Verification items for this drawing (mm, ordinates from the low corner). Round coordinates to 2 decimals unless told otherwise and drop trailing zeros. Loops run counter-clockwise (first coordinate to the right, second up) from the corner with the lowest first, then second, coordinate; pieces in that order, holes last. Notation, with made-up numbers: M -13,75 L -2,75 A24 ccw -2,104 Z; hole C -22,33.25 d11. An arc over 180 degrees is marked long. Write item = value, one per line.
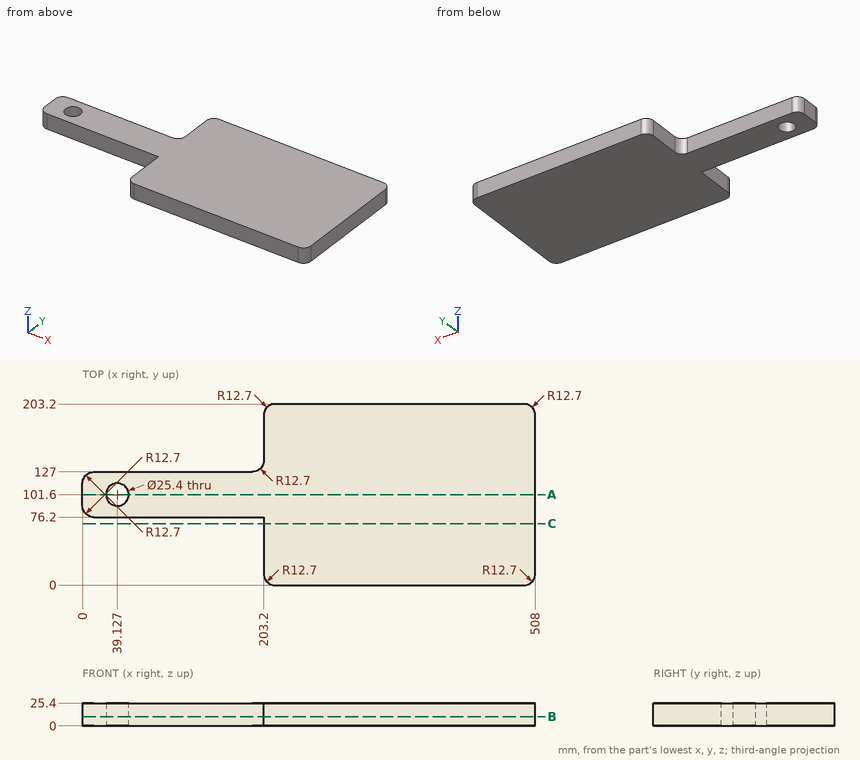
(1) Depth check by flat-ended pin: pin 1 Ø5 at (y, z) = (158, 13.5) entering from -X; pin 2 Ø3 at (x, z) = (148, 6) entering from -Y. Enter the tip coordinate at first touch or a pass-through.
Result set:
pin_1 = 203.2
pin_2 = 76.2
(2) Sectioned sample at B-B on z = 10.25. Record the cut outline in (x, y), then the cut area to 3 significant figures.
Result set:
outline = M 0,88.9 A12.7 ccw 12.7,76.2 L 203.2,76.2 L 203.2,12.7 A12.7 ccw 215.9,0 L 495.3,0 A12.7 ccw 508,12.7 L 508,190.5 A12.7 ccw 495.3,203.2 L 215.9,203.2 A12.7 ccw 203.2,190.5 L 203.2,139.7 A12.7 cw 190.5,127 L 12.7,127 A12.7 ccw 0,114.3 Z; hole C 39.13,101.6 d25.4
area = 71,600 mm2
(3) Sectioned sample at A-A on y = 101.6. Record the cut outline in (x, z), then the cut area to 3 significant figures.
Result set:
outline = M 0,0 L 26.43,0 L 26.43,25.4 L 0,25.4 Z; M 51.83,0 L 508,0 L 508,25.4 L 51.83,25.4 Z
area = 12,300 mm2
(4) Material ranges on line 1 along X through (y, z) = (22.5, 21); line 2 along Y through (x, z) = (177, 6.25); line 3 along X through (y, z) = (195, 12.5) (1 decimal), recorded low to high. Write a range as from..to.
Result set:
line_1 = 203.2..508
line_2 = 76.2..127
line_3 = 204..507.2
(5) Sectioned sample at C-C on y = 69. Record the cut outline in (x, z).
Result set:
outline = M 203.2,0 L 508,0 L 508,25.4 L 203.2,25.4 Z
